Can you work these out from the model? Positions are in its coordinate system, mm. A direction names the side the tool comes from. Round coordinates to 2 decimals unless told otherwise and drop trailing zeros. Write each loop counter-clockwise with the first axis right and the second up, starting at its lowest first coordinate (ties: lowest second). Pieces come first, ordered by that corner, then holes.
Q1. I'm going to push flat-ended pins straight in: pin 1 Ø8 at (x, z) = (6.5, 12.5) entering from -Y; pin 2 Ø0.8 at (y, z) = (-2, 29.5) entering from -X; pin 3 Ø8 at (y, z) = (-4, 25) entering from -X; pin 4 Ø8.5 at (x, z) = (0, 13) entering from +Y. Where does each tip first touch, or does it pass through?
Q2. For faces 1 (the flat face through (0, -5, 29)), 2 (the flat face through (-9.644, 2.149, 15.036)), 3 (the flat face through (9.673, 2.2, 15.036)), which set-ups out of +Z, -Z, +X, -X, +Y, -Y let a thin tool reach every point of the face, with its end or its side?
Q3. If we section it at A-A (y = -1.5): Please give me the cut outline in (x, z), plus the area to 3 significant figures.
Q4. We'd pull the mould along Z, two halves only. Please class faces 4 (the cylindrical face through (0.143, 1.891, 9.753)), 5 (the cylindrical face through (10.124, -4.238, -3.399)), 6 (the flat face through (0, -14.248, -1)): +Z half, -Z half, draft (parallel to the pull), parting line (faces both ways), or undercut.
Q5. If we section it at B-B (x = 0): Please give me the cut outline in (y, z), plus the area to 3 significant figures.
Q6. Please list where these lines run through material, in increasing order: line 1 along Z through (x, y) = (0, 2.5); line 2 along Z through (x, y) = (3.25, -8.5); line 3 along X through (y, z) = (1.5, 13).
Q7. If we section it at D-D (y = 2.5): Please give me the cut outline in (x, z), plus the area to 3 significant figures.
Q8. If we section it at C-C (z = 13): Please give me the cut outline in (x, y), plus the area to 3 significant figures.
from build123d import *

# Parameters (mm, degrees)
BOSS_EXTRUDE1_DEPTH     = 30.5
BOSS_EXTRUDE2_DEPTH     = 4
CUT_EXTRUDE1_DEPTH      = 36.321701763
CUT_EXTRUDE1_DEPTH_BACK = 36.321701763
SKETCH3_R               = 3.25
BOSS_EXTRUDE3_DEPTH     = 3
FILLET2_R               = 2


with BuildPart() as part:
    # Sketch1 → Boss-Extrude1 (new body)
    with BuildSketch(Plane.XY):
        with BuildLine():
            Line((-8.621574968, 0.348529625), (-10.694763671, 4))
            Line((-10.694763671, 4), (10.694763671, 4))
            Line((10.694763671, 4), (8.621574968, 0.348529625))
            ThreePointArc((8.621574968, 0.348529625), (7.717960529, -0.481070004), (6.5, -0.627106808))
            ThreePointArc((6.5, -0.627106808), (0, 0), (-6.5, -0.627106808))
            ThreePointArc((-6.5, -0.627106808), (-7.717960529, -0.481070004), (-8.621574968, 0.348529625))
        make_face()
    extrude(amount=BOSS_EXTRUDE1_DEPTH)

    # Sketch2 → Boss-Extrude2 (add)
    with BuildSketch(Plane.XY):
        with BuildLine():
            Line((10.694763671, 4), (10.694763671, -12.24761894))
            ThreePointArc((10.694763671, -12.24761894), (10.108977233, -13.661832502), (8.694763671, -14.24761894))
            Line((8.694763671, -14.24761894), (-8.694763671, -14.24761894))
            ThreePointArc((-8.694763671, -14.24761894), (-10.108977233, -13.661832502), (-10.694763671, -12.24761894))
            Line((-10.694763671, -12.24761894), (-10.694763671, 4))
            Line((-10.694763671, 4), (10.694763671, 4))
        make_face()
    extrude(amount=-BOSS_EXTRUDE2_DEPTH)

    # Sketch3 → Cut-Extrude1 (cut, two sides: drawn at the far end of the back side and taken through both)
    with BuildSketch(Plane(origin=(0, 0, 0), x_dir=(1, 0, 0), z_dir=(0, 1, 0)).offset(-CUT_EXTRUDE1_DEPTH_BACK)):
        with Locations(Location((0, -13, 0), (0, 0, 270))):
            Circle(SKETCH3_R)
    extrude(amount=CUT_EXTRUDE1_DEPTH + CUT_EXTRUDE1_DEPTH_BACK, mode=Mode.SUBTRACT)

    # Sketch4 → Boss-Extrude3 (add)
    with BuildSketch(Plane.XY.offset(30.5)):
        with BuildLine():
            Line((-5, 4), (5, 4))
            Line((5, 4), (5, -3))
            ThreePointArc((5, -3), (4.414213562, -4.414213562), (3, -5))
            Line((3, -5), (-3, -5))
            ThreePointArc((-3, -5), (-4.414213562, -4.414213562), (-5, -3))
            Line((-5, -3), (-5, 4))
        make_face()
    extrude(amount=-BOSS_EXTRUDE3_DEPTH)

    # Fillet2
    fillet2_edges = [part.edges().sort_by_distance(p)[0] for p in [
        (-10.108977233, -13.661832502, -4),
        (-10.694763671, -4.12380947, -4),
        (10.694763671, -4.12380947, -4),
        (10.108977233, -13.661832502, -4),
        (0, -14.24761894, -4),
    ]]
    fillet(fillet2_edges, radius=FILLET2_R)


solid = part.part
A:
1. pin 1: stops at y = -0.66
1. pin 2: stops at x = -5
1. pin 3: stops at x = -8.37
1. pin 4: stops at y = 4
2. face 1: +Z, +X, -X, -Y
2. face 2: +Z, -X, -Y
2. face 3: +Z, +X, -Y
3. outline: (-10.69, -2) arc R2 ccw to (-8.69, -4) - (8.69, -4) arc R2 ccw to (10.69, -2) - (10.69, 0) - (-10.69, 0) - close; (-5, 27.5) - (5, 27.5) - (5, 30.5) - (-5, 30.5) - close
3. area: 114 mm2
4. face 4: undercut
4. face 5: -Z half
4. face 6: draft
5. outline: (-14.25, -2) arc R2 ccw to (-12.25, -4) - (4, -4) - (4, 9.75) - (0, 9.75) - (0, 0) - (-14.25, 0) - close; (-5, 27.5) - (0, 27.5) - (0, 16.25) - (4, 16.25) - (4, 30.5) - (-5, 30.5) - close
5. area: 183 mm2
6. line 1: z = -4 to 9.75, 16.25 to 30.5
6. line 2: z = -4 to 0
6. line 3: x = -9.28 to -3.25, 3.25 to 9.28
7. outline: (-10.69, -2) arc R2 ccw to (-8.69, -4) - (8.69, -4) arc R2 ccw to (10.69, -2) - (10.69, 0) - (9.84, 0) - (9.84, 30.5) - (-9.84, 30.5) - (-9.84, 0) - (-10.69, 0) - close; hole circle Ø6.5 at (0, 13)
7. area: 651 mm2
8. outline: (-10.69, 4) - (-8.62, 0.35) arc R2 ccw to (-6.5, -0.63) arc R34 cw to (-3.25, -0.16) - (-3.25, 4) - close; (3.25, -0.16) arc R34 cw to (6.5, -0.63) arc R2 ccw to (8.62, 0.35) - (10.69, 4) - (3.25, 4) - close
8. area: 54.7 mm2
